For this review, take the finished solid that the model builds, in its own axes (mm). Face numbers are marked on the shaded views. A direction names the side the tool comes from. Give positions to 0.01 mm unless a question says otherwise; leave off trailing zeros. Write each loop counter-clockwise with the first axis right and the second up, starting at its lowest first coordinate (ties: lowest second). Pieces come first, ordered by that corner, then holes. Notation, with made-up numbers: M 40,65.25 L 52,65.25 A21 ccw 52,72.25 Z; hole C 59,-25.5 d3. An arc over 180 degrees is marked long. Answer as a JSON object with one key per item and string values. Group by question number.
```python
from build123d import *

# Parameters (mm, degrees)
SKETCH1_R           = 63.5
BOSS_EXTRUDE1_DEPTH = 12.7
SKETCH7_R           = 2.54
CUT_EXTRUDE2_DEPTH  = 91.696141042
CUT_EXTRUDE3_DEPTH  = 91.696141042
SHELL1_T            = -2.54


with BuildPart() as part:
    # Sketch1 → Boss-Extrude1 (new body)
    with BuildSketch(Plane(origin=(0, 0, 0), x_dir=(1, 0, 0), z_dir=(0, 1, 0))):
        with Locations(Location((0, 0, 0), (0, 0, 270))):
            Circle(SKETCH1_R)
    extrude(amount=-BOSS_EXTRUDE1_DEPTH)

    # Sketch7 → Cut-Extrude2 (cut, through all)
    with BuildSketch(Plane(origin=(0, 0, 0), x_dir=(1, 0, 0), z_dir=(0, 1, 0))):
        with Locations(Location((19.563011922, -13.687656502, 0), (0, 0, 270))):
            Circle(SKETCH7_R)
        with Locations(Location((21.635364211, 10.098237048, 0), (0, 0, 270))):
            Circle(SKETCH7_R)
        with Locations(Location((2.072352288, 23.78589355, 0), (0, 0, 270))):
            Circle(SKETCH7_R)
        with Locations(Location((-19.563011922, 13.687656502, 0), (0, 0, 270))):
            Circle(SKETCH7_R)
        with Locations(Location((-21.635364211, -10.098237048, 0), (0, 0, 270))):
            Circle(SKETCH7_R)
        with Locations(Location((-2.072352288, -23.78589355, 0), (0, 0, 270))):
            Circle(SKETCH7_R)
    extrude(amount=-CUT_EXTRUDE2_DEPTH, mode=Mode.SUBTRACT)

    # Sketch8 → Cut-Extrude3 (cut, through all)
    with BuildSketch(Plane(origin=(0, 0, 0), x_dir=(1, 0, 0), z_dir=(0, 1, 0))):
        Polygon((-6.702144956, -3.150433197), (-0.622717296, -7.37944439), (6.079427659, -4.229011193), (6.702144956, 3.150433197), (0.622717296, 7.37944439), (-6.079427659, 4.229011193), align=None)
    extrude(amount=-CUT_EXTRUDE3_DEPTH, mode=Mode.SUBTRACT)

    # Shell1
    shell1_openings = [part.faces().sort_by_distance(p)[0] for p in [
        (-2.072352288, -6.35, 21.24589355),
        (19.563011922, -6.35, 11.147656502),
        (0, 0, -61.703948776),
        (-21.635364211, -6.35, 7.558237048),
        (-19.563011922, -6.35, -16.227656502),
        (2.072352288, -6.35, -26.32589355),
        (21.635364211, -6.35, -12.638237048),
        (-6.390786307, -6.35, -0.539288998),
        (-2.728355181, -6.35, -5.804227791),
        (3.662431126, -6.35, -5.264938793),
        (6.390786307, -6.35, 0.539288998),
        (2.728355181, -6.35, 5.804227791),
        (-3.662431126, -6.35, 5.264938793),
    ]]
    offset(amount=SHELL1_T, openings=shell1_openings, kind=Kind.INTERSECTION)


solid = part.part
```
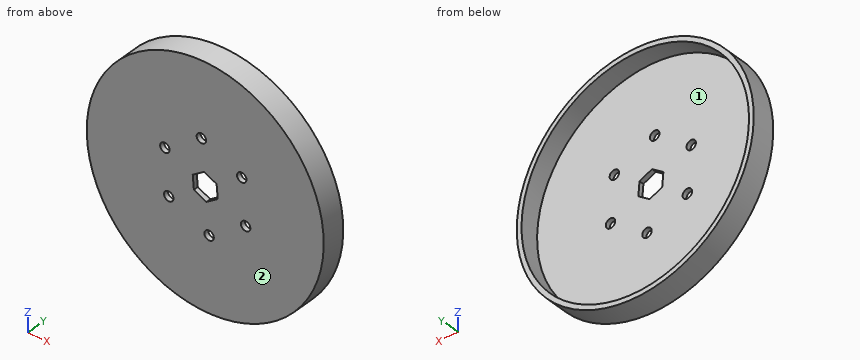
Item 1: To check wall thickness, follow probe 1 along Z at (x, y) = (-21.5, -10.5); probe 2 along Y at (x, z) = (-17.5, 6); probe 3 along X at (y, z) = (-6.75, 0.5). State the ranges of each line that lie inside material, in increasing order.
Item 2: Consider section A-A (z = 0). Give the boundary of the cut face in (x, y), plus the area to 3 significant figures.
Item 3: Machinability: for the marked faces 1 and 2, which of the approach directions +Z, -Z, +X, -X, +Y, -Y give a long, thin tool a straight path to every point of the face, cutting with its end or side? Answer none if there is none.
Item 4: Consider section D-D (z = -51.5). Give the boundary of the cut face in (x, y).
Item 5: Insertion check: P1, Ø4.5, axis at x = -19.56, z = -13.69, coming from the -Y side; P2, Ø10, axis at x = 40, z = -5.5, coming from the +Y side; P3, Ø1, axis at x = -10.5, y = -2, coming from the -Z side; P4, Ø1.5, axis at y = -5.5, z = -13.5, coming from the +X side. Each pin has a flat end and moves straight along its axis. Give the tip position at first contact, or say it passes through.
Item 6: Consider section C-C (y = -7.5). Give the boundary of the cut face in (x, z).
Item 7: Consider section B-B (x = 34). Give the boundary of the cut face in (y, z).
Result set:
{
 "1": {"probe 1": "z = -59.75 to -15.33, -12.04 to 7.56, 12.63 to 59.75", "probe 2": "y = -12.7 to -10.16", "probe 3": "x = -63.5 to -60.96, 60.96 to 63.5"},
 "2": {"outline": "M -63.5,-12.7 L -6.44,-12.7 L -6.44,-10.16 L -60.96,-10.16 L -60.96,0 L -63.5,0 Z; M 6.44,-12.7 L 63.5,-12.7 L 63.5,0 L 60.96,0 L 60.96,-10.16 L 6.44,-10.16 Z", "area": "341 mm^2"},
 "3": {"face 1": "+Y", "face 2": "+Z, -Z, +X, -X, -Y"},
 "4": {"outline": "M -37.15,-12.7 L 37.15,-12.7 L 37.15,0 L 32.62,0 L 32.62,-10.16 L -32.62,-10.16 L -32.62,0 L -37.15,0 Z"},
 "5": {"P1": "passes through", "P2": "stops at y = -10.16", "P3": "stops at z = -62.71", "P4": "stops at x = 62.21"},
 "6": {"outline": "C 0,0 d127; hole C 0,0 d121.92"},
 "7": {"outline": "M -12.7,-53.63 L 0,-53.63 L 0,-50.6 L -10.16,-50.6 L -10.16,50.6 L 0,50.6 L 0,53.63 L -12.7,53.63 Z"}
}
